Geometry: final body of the model. Coordinates: model frame, mm. A direction names the side the tool comes from. Round coordinates to 2 decimals unless told otherwise and drop trailing zeros. Loops run counter-clockwise (first coordinate to the right, second up) from the corner with the lowest first, then second, coordinate; pieces in that order, holes last. Notation, with made-up numbers: (4.5, 13) -> (43.5, 13) arc R29 cw to (43.5, 51) -> close; hole circle Ø6 at (-34.5, 68.5). An arc over 180 degrees is marked (long way). Answer in a Markdown table with one row per item.
Autodesk Inventor part; units mm, degrees
ref_plane "YZ Plane" through (0, 0, 0) normal (1, 0, 0) x (0, 1, 0)
ref_plane "XZ Plane" through (0, 0, 0) normal (0, 1, 0) x (-1, 0, 0)
ref_plane "XY Plane" through (0, 0, 0) normal (0, 0, 1) x (1, 0, 0)
sketch "Sketch1" plane through (0, 0, 0) normal (0, 1, 0) x (-1, 0, 0)
  line L0 (8.95, -4.25) -> (-8.95, -4.25)
  line L1 (-8.95, -4.25) -> (-8.95, 4.25)
  line L2 (-8.95, 4.25) -> (8.95, 4.25)
  line L3 (8.95, 4.25) -> (8.95, -4.25)
  point P0 (0, 0)
  point P1 (0, -4.25)
  point P2 (-8.95, 0)
  dimension "d0" = 17.9
  dimension "d1" = 8.5
extrude "Extrusion1" add sketch "Sketch1" along normal blind 7.9
sketch "Sketch2" plane through (0, 0, 0) normal (0, -1, 0) x (1, 0, 0)
  line L0 (-8.95, 4.25) -> (8.95, 4.25)
  line L1 (-8.95, 4.25) -> (-5.95, 4.25)
  line L2 (-5.95, 4.25) -> (-5.95, -4.25)
  line L3 (-5.95, -4.25) -> (-8.95, -4.25)
  line L4 (-8.95, -4.25) -> (-8.95, 4.25)
  line L5 (8.95, 4.25) -> (5.95, 4.25)
  line L6 (5.95, 4.25) -> (5.95, -4.25)
  line L7 (5.95, -4.25) -> (8.95, -4.25)
  line L8 (8.95, -4.25) -> (8.95, 4.25)
  line L9 (8.95, -4.25) -> (-8.95, -4.25)
  line L10 (-5.95, 4.25) -> (5.95, 4.25)
  line L11 (5.95, 4.25) -> (5.95, 3.5)
  line L12 (5.95, 3.5) -> (-5.95, 3.5)
  line L13 (-5.95, 3.5) -> (-5.95, 4.25)
  line L14 (-5.95, -4.25) -> (5.95, -4.25)
  line L15 (5.95, -4.25) -> (5.95, -3.5)
  line L16 (5.95, -3.5) -> (-5.95, -3.5)
  line L17 (-5.95, -3.5) -> (-5.95, -4.25)
  point P0 (0, 0)
  point P1 (-5.95, 3.5)
  dimension "d4" = 3
  dimension "d5" = 3
  dimension "d6" = 0.75
extrude "Extrusion2" cut sketch "Sketch2" against normal blind 1 contours L0 L2 L3 L4 | L0 L8 L7 L6 | L12 L6 L16 L2
sketch "Sketch3" plane through (0, 0, 0) normal (0, 1, 0) x (-1, 0, 0)
  line L0 (9.5, 2.75) -> (7.7, 2.75)
  line L1 (7.7, 2.75) -> (7.7, 2.25)
  line L2 (7.7, 2.25) -> (9.5, 2.25)
  line L3 (9.5, 2.25) -> (9.5, 2.75)
  line L4 (9.5, -2.25) -> (7.7, -2.25)
  line L5 (7.7, -2.25) -> (7.7, -2.75)
  line L6 (7.7, -2.75) -> (9.5, -2.75)
  line L7 (9.5, -2.75) -> (9.5, -2.25)
  line L8 (9.5, 2.5) -> (9.5, -2.5) construction
  line L9 (-7.7, 3.3) -> (-9.5, 3.3)
  line L10 (-9.5, 3.3) -> (-9.5, 2.8)
  line L11 (-9.5, 2.8) -> (-7.7, 2.8)
  line L12 (-7.7, 2.8) -> (-7.7, 3.3)
  line L13 (-7.7, -2.8) -> (-9.5, -2.8)
  line L14 (-9.5, -2.8) -> (-9.5, -3.3)
  line L15 (-9.5, -3.3) -> (-7.7, -3.3)
  line L16 (-7.7, -3.3) -> (-7.7, -2.8)
  line L17 (-9.5, 3.05) -> (-9.5, -3.05) construction
  line L18 (9.5, 0) -> (-9.5, 0) construction
  point P0 (0, 0)
  point P1 (8.6, -2.25)
  point P2 (8.6, 2.25)
  point P3 (-8.6, -2.8)
  point P4 (-8.6, 2.8)
  point P5 (0, 0)
  dimension "d9" = 0.5
  dimension "d10" = 1.8
  dimension "d11" = 0.5
  dimension "d12" = 1.8
  dimension "d13" = 5
  dimension "d14" = 0.5
  dimension "d15" = 1.8
  dimension "d16" = 0.5
  dimension "d17" = 1.8
  dimension "d19" = 6.1
  dimension "d20" = 19
extrude "Extrusion3" add sketch "Sketch3" along normal blind 1
sketch "Sketch4" plane through (0, 7.9, 0) normal (0, 1, 0) x (1, 0, 0)
  circle A0 centre (-7, -2.5) radius 0.8343
  line L0 (-7, -1.6657) -> (-7, -3.3343)
  point P0 (0, 0)
  dimension "d23" = 7
  dimension "d24" = 2.5
revolve "Revolution1" cut sketch "Sketch4" angle 360 about axis through (-7, 7.9, 1.6657) along (0, 0, 1) picked at (-6.7647, -2.2895) contours A0 L0
properties part number "ZS1052_S_HT"
Item 1: Pin query (flat end, axial travel): pin 1 Ø3.5 at (y, z) = (3, 1) entering from -X; pin 2 Ø1.1 at (x, y) = (8, 0.5) entering from -Z; pin 3 Ø0.6 at (y, z) = (0.5, 3.5) entering from -X; pin 4 Ø0.8 at (x, y) = (8.5, 0.5) entering from +Z. Return the tip coordinate at first contact, or that it passes through.
Answer:
| item | result |
|---|---|
| pin 1 | stops at x = -8.95 |
| pin 2 | stops at z = -4.25 |
| pin 3 | stops at x = -5.95 |
| pin 4 | stops at z = 3.3 |
Item 2: Cut plane D-D (z = -2). Output: boundary loops of the cut face in (x, y).
Answer:
| item | result |
|---|---|
| outline | (-8.95, 1) -> (8.95, 1) -> (8.95, 7.9) -> (-8.95, 7.9) -> close |
Item 3: Cut plane C-C (y = 4.75). Output: boundary loops of the cut face in (x, z).
Answer:
| item | result |
|---|---|
| outline | (-8.95, -4.25) -> (8.95, -4.25) -> (8.95, 4.25) -> (-8.95, 4.25) -> close |
Item 4: Reachability of faces 1 (the face through (-8.6, 0.5, -2.25)), 2 (the face through (0, 4, 4.25)), 3 (the face through (0, 4, -4.25)), 4 (the face through (8.6, 0.5, -3.3)), 5 (the face through (-8.6, 0.5, 2.75)) from +Z, -Z, +X, -X, +Y, -Y: full face, straight path, thin tool, end or side. Return the list, or none.
Answer:
| item | result |
|---|---|
| face 1 | +X, -X, -Y |
| face 2 | +Z, +X, -X, +Y, -Y |
| face 3 | -Z, +X, -X, +Y, -Y |
| face 4 | -Z, +X, -X, -Y |
| face 5 | +Z, +X, -X, -Y |
Item 5: Draft query along Z for faces 6 (the face through (8.6, 0.5, 3.3)), 7 (the face through (0, 7.9, 0)), 8 (the face through (8.6, 0.5, -2.8)). Return one class per face: pulls with the +Z half, pulls with the -Z half, needs draft (parallel to the pull), parting line crosses it, or undercut.
Answer:
| item | result |
|---|---|
| face 6 | pulls with the +Z half |
| face 7 | needs draft |
| face 8 | undercut |
Item 6: Cut plane A-A (x = -5.5). Output: boundary loops of the cut face in (y, z).
Answer:
| item | result |
|---|---|
| outline | (0, -4.25) -> (7.9, -4.25) -> (7.9, 4.25) -> (0, 4.25) -> (0, 3.5) -> (1, 3.5) -> (1, -3.5) -> (0, -3.5) -> close |
Item 7: Cut plane B-B (z = 3). Output: boundary loops of the cut face in (x, y).
Answer:
| item | result |
|---|---|
| outline | (-8.95, 1) -> (7.7, 1) -> (7.7, 0) -> (9.5, 0) -> (9.5, 1) -> (8.95, 1) -> (8.95, 7.9) -> (-6.33, 7.9) arc R0.67 cw to (-7.67, 7.9) -> (-8.95, 7.9) -> close |
Item 8: Line query: probe 1 along X at (y, z) = (3, 3.5); probe 2 along Y at (x, z) = (-5.75, -2.75). Output: solid intervals per line, ascending. Write a range as [from, to].
Answer:
| item | result |
|---|---|
| probe 1 | x = [-8.95, 8.95] |
| probe 2 | y = [1, 7.9] |
